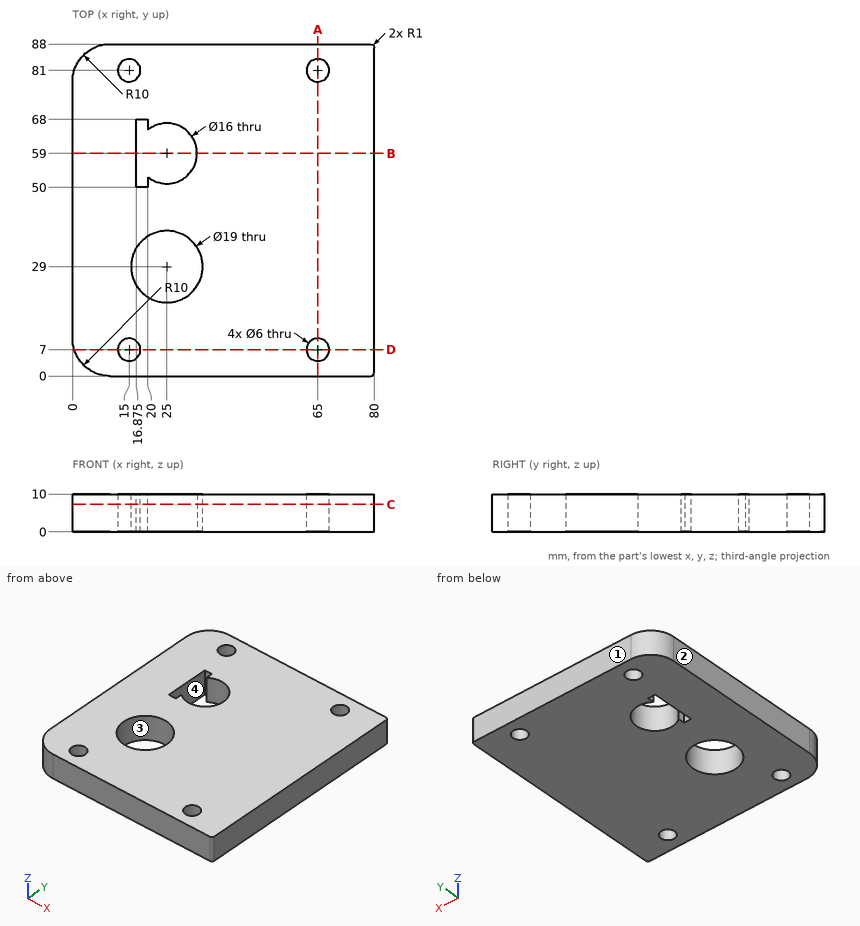
Input: dimensioned drawing with shaded views. Units: mm. Origin: part minimum x, y, z. Round coordinates to 2 decimals unless told otherwise and drop trailing zeros. Loops run counter-clockwise (first coordinate to the right, second up) from the corner with the lowest first, then second, coordinate; pieces in that order, holes last. Notation, with made-up numbers: M 73,21 L 106,21 A6 ccw 106,28 Z; hole C 37,87.5 d8. An arc over 180 degrees is marked long. Return JSON: item names as keys, results as strings. Group by question number.
1. Material intervals for line 1 along Y through (x, z) = (65, 6.75); line 2 along Y through (x, z) = (25, 2.5); line 3 along X through (y, z) = (59, 6.75) (3 decimals), sorted ascending. Write a range as from..to.
2. Section query B-B on y = 59. Output: boundary loops of the cut face in (x, z) (3 decimals).
3. Mould query, pull axis Y, two halves, no side actions, for the marked faces 1, 2, 3 and 4. Classes: released by +Y, released by -Y, zero draft, split by the parting line, or undercut.
4. Section query D-D on y = 7. Output: boundary loops of the cut face in (x, z).
5. Section query A-A on x = 65. Output: boundary loops of the cut face in (y, z).
6. Section query C-C on z = 7.25. Output: boundary loops of the cut face in (x, y) (3 decimals).
7. Pin query (flat end, axial travel): pin 1 (5 mm diameter, centred on x = 15, y = 7, fed in from +Z). Return the tip coordinate at first contact, or that it passes through.
Checks:
{
 "1": {"line 1": "y = 0..4, 10..78, 84..88", "line 2": "y = 0..19.5, 38.5..51, 67..88", "line 3": "x = 0..16.875, 33..80"},
 "2": {"outline": "M 0,0 L 16.875,0 L 16.875,10 L 0,10 Z; M 33,0 L 80,0 L 80,10 L 33,10 Z"},
 "3": {"face 1": "released by +Y", "face 2": "zero draft", "face 3": "undercut", "face 4": "undercut"},
 "4": {"outline": "M 0.46,0 L 12,0 L 12,10 L 0.46,10 Z; M 18,0 L 62,0 L 62,10 L 18,10 Z; M 68,0 L 80,0 L 80,10 L 68,10 Z"},
 "5": {"outline": "M 0,0 L 4,0 L 4,10 L 0,10 Z; M 10,0 L 78,0 L 78,10 L 10,10 Z; M 84,0 L 88,0 L 88,10 L 84,10 Z"},
 "6": {"outline": "M 0,10 A10 ccw 10,0 L 79,0 A1 ccw 80,1 L 80,87 A1 ccw 79,88 L 10,88 A10 ccw 0,78 Z; hole C 15,7 d6; hole C 15,81 d6; hole C 25,29 d19; hole M 16.875,50 L 20,50 L 20,52.755 A8 ccw long 20,65.245 L 20,68 L 16.875,68 Z; hole C 65,7 d6; hole C 65,81 d6"},
 "7": {"pin 1": "passes through"}
}
